from build123d import *

# Parameters (mm, degrees)
BOSS_EXTRUDE1_DEPTH = 4
BOSS_EXTRUDE2_DEPTH = 3
SKETCH4_R           = 1.75
CUT_EXTRUDE1_DEPTH  = 8
SKETCH5_R           = 4.25
CUT_EXTRUDE2_DEPTH  = 4


with BuildPart() as part:
    # Sketch1 → Boss-Extrude1 (new body)
    with BuildSketch(Plane.XY):
        with BuildLine():
            Line((0, 79), (0, 69))
            ThreePointArc((0, 69), (23.599389889, 64.838790834), (44.352345068, 52.857066575))
            Line((44.352345068, 52.857066575), (50.780221165, 60.517511006))
            ThreePointArc((50.780221165, 60.517511006), (27.019591323, 74.235717042), (0, 79))
        make_face()
    extrude(amount=BOSS_EXTRUDE1_DEPTH)

    # Sketch2 → Boss-Extrude2 (add)
    with BuildSketch(Plane.XY.offset(4)):
        with BuildLine():
            Line((44.352345068, 52.857066575), (53.351371604, 63.581688779))
            ThreePointArc((53.351371604, 63.581688779), (28.387671896, 77.994487525), (0, 83))
            Line((0, 83), (0, 69))
            ThreePointArc((0, 69), (23.599389889, 64.838790834), (44.352345068, 52.857066575))
        make_face()
    extrude(amount=BOSS_EXTRUDE2_DEPTH)

    # Sketch4 → Cut-Extrude1 (cut, through all)
    with BuildSketch(Plane.XY.offset(7)):
        with Locations((12.849965147, 72.875773723)):
            Circle(SKETCH4_R)
        with Locations((37, 64.08587988)):
            Circle(SKETCH4_R)
    extrude(amount=-CUT_EXTRUDE1_DEPTH, mode=Mode.SUBTRACT)

    # Sketch5 → Cut-Extrude2 (cut)
    with BuildSketch(Plane(origin=(0, 0, 7), x_dir=(-1, 0, 0), z_dir=(0, 0, -1))):
        with Locations((-37, 64.08587988)):
            Circle(SKETCH5_R)
        with Locations((-12.849965147, 72.875773723)):
            Circle(SKETCH5_R)
    extrude(amount=CUT_EXTRUDE2_DEPTH, mode=Mode.SUBTRACT)


solid = part.part
Design review of the part built by this model. Coordinates are the model's own, in mm. A direction names the side the tool comes from. Give positions to 0.01 mm unless a question says otherwise; leave off trailing zeros. Loops run counter-clockwise (first coordinate to the right, second up) from the corner with the lowest first, then second, coordinate; pieces in that order, holes last. Notation, with made-up numbers: (26.5, 28) -> (40.5, 28) arc R23 ccw to (40.5, 46) -> close; hole circle Ø8 at (42.25, -36.75). An arc over 180 degrees is marked (long way). One line per question, with ' | ' between items. Start each with the question number.
(1) We need section C-C (x = 19). State the section outline as (y, z) points, and give its area (3 significant figures).
(2) For faces 1 (the face through (12, 71, 3)), 2 (the face through (26, 71, 7)), 3 (the face through (27.382, 74.103, 1.972)), list the 3-axis set-ups (+Z, -Z, +X, -X, +Y, -Y) from which the entire face can be reached by the end or side of a thin tool; tool diameter is ignored.
(3) We need section B-B (x = 37). State the section outline as (y, z) points, and give its area (3 significant figures).
(4) For line 1 (Z direction, x = 34, y = 65.5); line 2 (Y direction, x = 11, z = 4.25); line 3 (X direction, y = 62, z = 6.5), list the stretches that pass through material, from the lowest coordinate up.
(5) Insertion check: P1, Ø12, axis at x = 12, y = 72.5, coming from the -Z side; P2, Ø7.5, axis at x = 37, y = 64.09, coming from the +Z side; P3, Ø1.5, axis at y = 64, z = 1, coming from the +X side; P4, Ø1.5, axis at x = 34.5, z = 3.5, coming from the +Y side. Each pin has a flat end and moves straight along its axis. Give the tip position at first contact, or say it passes through.
(6) We need section A-A (y = 73.5). State the section outline as (x, z) points, and give its area (3 significant figures).
(7) We need section D-D (y = 78). State the section outline as (x, z) points.
The answers:
1) outline: (66.33, 0) -> (76.68, 0) -> (76.68, 4) -> (80.8, 4) -> (80.8, 7) -> (66.33, 7) -> close | area: 84.8 mm^2
2) face 1: +Z | face 2: +Z, +X, -X, +Y, -Y | face 3: -Z, +X, +Y
3) outline: (58.24, 0) -> (62.34, 0) -> (62.34, 3) -> (59.84, 3) -> (59.84, 7) -> (58.24, 7) -> close; (65.84, 0) -> (69.8, 0) -> (69.8, 4) -> (74.3, 4) -> (74.3, 7) -> (68.34, 7) -> (68.34, 3) -> (65.84, 3) -> close | area: 49.9 mm^2
4) line 1: z = 0 to 3 | line 2: y = 68.12 to 69.05, 76.7 to 82.27 | line 3: x = 30.28 to 33.3, 40.7 to 52.02
5) P1: stops at z = 0 | P2: stops at z = 3 | P3: stops at x = 47.33 | P4: stops at y = 75.74
6) outline: (0, 0) -> (11.22, 0) -> (11.22, 3) -> (8.65, 3) -> (8.65, 7) -> (0, 7) -> close; (14.48, 0) -> (28.96, 0) -> (28.96, 4) -> (38.56, 4) -> (38.56, 7) -> (17.05, 7) -> (17.05, 3) -> (14.48, 3) -> close | area: 188 mm^2
7) outline: (0, 0) -> (12.53, 0) -> (12.53, 4) -> (28.37, 4) -> (28.37, 7) -> (0, 7) -> close
